Input: part model. Units: mm. Frame: model coordinates. Round coordinates to 2 decimals unless told otherwise and drop trailing zeros. Loops run counter-clockwise (first coordinate to the right, second up) from the corner with the lowest first, then second, coordinate; pieces in that order, holes last. Notation, with made-up numbers: (48, -25) - (104, -25) arc R21 ccw to (104, 12) - close; hole circle Ø10 at (-22, 25). An arc over 180 degrees is marked (long way). One line per question, with ' | ' between items. Start each with the question number.
Item 1: Draft query along X for faces 1 (the face through (34.292, 0, 7)), 2 (the face through (-36.6, 0.3, 3.6)), 3 (the face through (-6, 1, 15)). Return one class per face: pulls with the +X half, pulls with the -X half, needs draft (parallel to the pull), parting line crosses it, or undercut.
Item 2: Section A-A, the plane z = 7.5. Return loops of the section in (x, y).
Item 3: Section B-B, the plane y = 19. Return loops of the section in (x, z), plus the area to 3 significant figures.
Item 4: Material intervals for line 1 along X through (y, z) = (8, 6); line 2 along X through (y, z) = (-17, 9.5); line 3 along Z through (x, y) = (26, 0), sorted ascending.
Item 5: First-contact query: pin 1 (6.5 mm diameter, centred on x = -35.71, z = 7.5, fed in from +Y). Flat tip, straight axial feed; report the tip coordinate or a pass-through.
```python
from build123d import *

# Parameters (mm, degrees)
F0_W     = 80
F0_H     = 50
F1_DEPTH = 15
F2_R     = 4
F3_DEPTH = 50


with BuildPart() as f1:
    # F0 (on Top) → F1 (new body)
    with BuildSketch(Plane.XY):
        with Locations((-5.707638, 0.697194)):
            Rectangle(F0_W, F0_H)
    extrude(amount=F1_DEPTH)

    # F2 (on face) → F3 (cut)
    with BuildSketch(Plane.XZ.offset(24.302806)):
        with Locations((-35.707638, 7.5)):
            Circle(F2_R)
        with Locations((24.292362, 7.5)):
            Circle(F2_R)
    extrude(amount=-F3_DEPTH, mode=Mode.SUBTRACT)


solid = f1.part
```
Return value:
1) face 1: pulls with the +X half | face 2: undercut | face 3: needs draft
2) outline: (-45.71, -24.3) - (-39.71, -24.3) - (-39.71, 25.7) - (-45.71, 25.7) - close; (-31.71, -24.3) - (20.29, -24.3) - (20.29, 25.7) - (-31.71, 25.7) - close; (28.29, -24.3) - (34.29, -24.3) - (34.29, 25.7) - (28.29, 25.7) - close
3) outline: (-45.71, 0) - (34.29, 0) - (34.29, 15) - (-45.71, 15) - close; hole circle Ø8 at (-35.71, 7.5); hole circle Ø8 at (24.29, 7.5) | area: 1,100 mm2
4) line 1: -45.71 to -39.42, -32 to 20.58, 28 to 34.29 | line 2: -45.71 to -39.17, -32.24 to 20.83, 27.76 to 34.29 | line 3: 0 to 3.88, 11.12 to 15
5) pin 1: through
